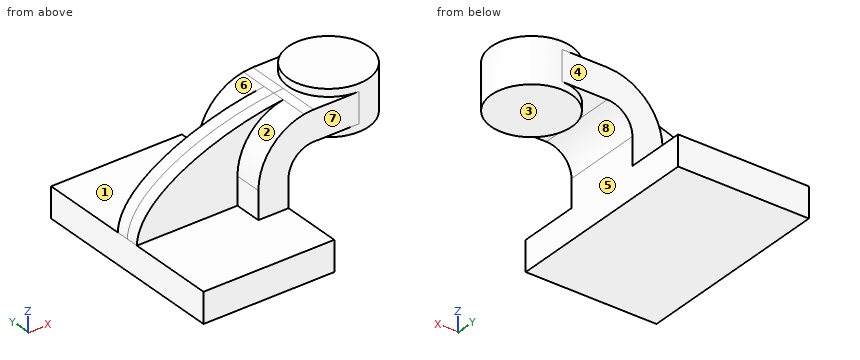
from build123d import *

# Parameters (mm, degrees)
F1_DEPTH = 63.5
F0_W     = 25.4
F0_H     = 19.05
F2_DEPTH = 25.4
F3_DEPTH = 7.9375


with BuildPart() as f1:
    # F0 (on Front) → F1 (new body, symmetric)
    with BuildSketch(Plane.XZ):
        Polygon((22.225, 9.525), (-41.275, 9.525), (-41.275, -9.525), (41.275, -9.525), (41.275, 9.525), align=None)
    extrude(amount=F1_DEPTH, both=True)

    # F0 (on Front) → F2 (join, symmetric)
    with BuildSketch(Plane.XZ):
        with BuildLine():
            Line((22.225, 27.0002), (22.225, 9.525))
            Line((22.225, 9.525), (41.275, 9.525))
            Line((41.275, 9.525), (41.275, 27.0002))
            ThreePointArc((41.275, 27.0002), (45.9246798487, 38.2255201513), (57.15, 42.8752))
            Line((57.15, 42.8752), (60.325, 42.8752))
            Line((60.325, 42.8752), (60.325, 61.9252))
            Line((60.325, 61.9252), (57.15, 61.9252))
            add(Edge.make_bspline(
                [(51.1376503086, 61.4037939429), (53.174688835, 61.6179457119), (55.1815563456, 61.7920560341), (57.15, 61.9252)],
                knots=[106.0980519126, 106.0980519126, 106.0980519126, 106.0980519126, 111.5045361635, 111.5045361635, 111.5045361635, 111.5045361635], degree=3))
            ThreePointArc((51.1376503086, 61.4037939429), (30.4129756894, 49.4698941682), (22.225, 27.0002))
        make_face()
        with Locations((73.025, 52.4002)):
            Rectangle(F0_W, F0_H)
    extrude(amount=F2_DEPTH, both=True)

    # F0 (on Front) → F3 (join, symmetric)
    with BuildSketch(Plane.XZ):
        with BuildLine():
            add(Edge.make_bspline(
                [(-41.275, 9.525), (-40.4321093733, 37.5783033458), (11.1623522611, 57.2012318992), (51.1376503086, 61.4037939429)],
                knots=[0, 0, 0, 0, 106.0980519126, 106.0980519126, 106.0980519126, 106.0980519126], degree=3))
            Line((-41.275, 9.525), (22.225, 9.525))
            Line((22.225, 9.525), (22.225, 27.0002))
            ThreePointArc((22.225, 27.0002), (30.4129756894, 49.4698941682), (51.1376503086, 61.4037939429))
        make_face()
    extrude(amount=F3_DEPTH, both=True)

    # F0 (on Front) → F4 (revolve)
    with BuildSketch(Plane.XZ):
        Polygon((85.725, 66.675), (85.725, 61.9252), (85.725, 42.8752), (85.725, 38.1), (111.125, 38.1), (111.125, 66.675), align=None)
    revolve(axis=Axis((85.725, 0, 54.7751), (0, 0, 1)))


solid = f1.part
Can you work these out from the model? Positions are in its coordinate system, mm. Face numbers are marked on the shaded views. A direction names the side the tool comes from. Coordinates: 2 decimals unless noted, no trailing zeros. Order: outer loops, then holes, each group sorted by start corner. A loop starts at its lowest first (then second) coordinate and runs counter-clockwise, first axis right, second up. Notation, with made-up numbers: (23, -16.5) -> (59, -16.5) arc R14 cw to (59, -11.5) -> close; hole circle Ø7 at (7, 12). An arc over 180 degrees is marked (long way). Use one line per item in the form item = value.
Q1. Imagine slicing it at B-B, the plane x = 91. List the corners of the cut face in (y, z) for me (3 decimals), then the cut area to 3 significant figures.
From the geometry:
outline = (-24.846, 38.1) -> (24.846, 38.1) -> (24.846, 66.675) -> (-24.846, 66.675) -> close
area = 1,420 mm²
Q2. We'd pull the mould along X, two halves only. Please class the marked faces 5, 6, 7 and 8: released by +X, released by -X, zero draft, split by the parting line, or undercut.
From the geometry:
face_5 = released by +X
face_6 = released by -X
face_7 = zero draft
face_8 = undercut
Q3. Will these pins go through, and if not, where does the flat tip stop? P1, Ø15.5, axis at x = 65, z = 34.5, coming from the +Y side; P2, Ø12, axis at y = -21, z = 51, coming from the -X side; P3, Ø12, axis at x = 63, z = 43.5, coming from the +Y side.
From the geometry:
P1 = 21.28
P2 = 27.22
P3 = 25.4
Q4. I need wall thicknesses on L1, parallel to Z at x = 13, y = -47.5 (3 decimals); L2, parallel to Y at x = 21, z = 50; L3, parallel to Y at x = 34, z = 42.5. Which ranges of each line are inside material? Lowest first, please.
From the geometry:
L1 = -9.525 to 9.525
L2 = -7.94 to 7.94
L3 = -25.4 to 25.4
Q5. Which directions (+Z, -Z, +X, -X, +Y, -Y) give clear straight access to the entire face, cutting with the end or side of a thin tool? Please do the marked faces 1, 2, 3 and 4.
From the geometry:
face_1 = +Z, -X, +Y
face_2 = +Z, -X, -Y
face_3 = -Z, +X, +Y, -Y
face_4 = +Z, +X, -X, +Y
Q6. Imagine slicing it at A-A, the plane y = 42. List the corners of the cut face in (x, z) for me (3 decimals).
From the geometry:
outline = (-41.275, -9.525) -> (41.275, -9.525) -> (41.275, 9.525) -> (-41.275, 9.525) -> close
